Build history of the part. All positions in model axes, mm. A direction names the side the tool comes from. Give positions to 0.01 mm unless a question says otherwise; leave off trailing zeros. Write each loop counter-clockwise with the first axis right and the second up, starting at its lowest first coordinate (ties: lowest second). Pieces come first, ordered by that corner, then holes. Notation, with made-up numbers: M 29.5,43 L 76.5,43 A15 cw 76.5,47 Z; hole C 60.25,4.5 d5. An arc over 180 degrees is marked long. Return JSON: item names as keys, results as strings. Group by question number.
Q1. Band-saw the part on A-A, the plane x = 12.7. Give the cut face in (y, z) (3 decimals).
Q2. Band-saw the part on B-B, the plane y = 25.4. Give the cut face in (x, z) (3 decimals).
Q3. Band-saw the part on D-D, the plane z = 0.25. Count the separate pieces of the cut face and the enclosed holes in it, then the cut area to 3 significant figures.
Q4. Pull direction Y, two halves, no side cores. Call faces 3 (the flat face through (14, 104.775, 0)), 4 (the flat face through (25.4, 66, 0)), 5 (the flat face through (32, 0, 0)): +Y half, -Y half, draft (parallel to the pull), parting line (faces both ways), or undercut.
Q5. Band-saw the part on C-C, the plane x = 38. Give the cut face in (y, z) (3 decimals).
Q6. Flat gauge pins, fed straight in: pin 1 Ø3 at (y, z) = (55.5, 1.5) entering from +X; pin 2 Ø1.9 at (x, z) = (39, 0) entering from +Y. Where does each tip first touch, or does it go through?
Q7. Wall check: probe 1 along Y at (x, z) = (12.7, 1.75) (3 decimals); probe 2 along Y at (x, z) = (50.8, -1.25); probe 3 along Y at (x, z) = (38.1, 1.25). Give the ranges that are in metal, low to high.
Q8. Tool access for faces 1 (the cylindrical face through (29.722, 79.774, -0.044)), 2 (the cylindrical face through (61.59, 1.81, 0.04)): list every direction of +Z, -Z, +X, -X, +Y, -Y with a clear straight run to the whole face (end or side of a thin tool).
from build123d import *

# Parameters (mm, degrees)
SKETCH1_R           = 2.4892
BOSS_EXTRUDE1_DEPTH = 3.175
LPATTERN1_START     = -3.175
LPATTERN1_OUTLINE_R = 2.4892
LPATTERN1_DEPTH     = 6.35
CUT_EXTRUDE1_DEPTH  = 123.679962198
FILLET1_R           = 6.35


# Read off the part's stored shape, not the designer's step: LPattern1
with BuildPart() as part:
    # Sketch1 → Boss-Extrude1 (new, symmetric)
    with BuildSketch(Plane.XY):
        Polygon((0, 0), (0, 104.775), (25.4, 104.775), (63.5, 50.8), (63.5, 0), align=None)
        with Locations((12.7, 85.725)):
            Circle(SKETCH1_R, mode=Mode.SUBTRACT)
        with Locations((12.7, 73.025)):
            Circle(SKETCH1_R, mode=Mode.SUBTRACT)
        with Locations((12.7, 12.7)):
            Circle(SKETCH1_R, mode=Mode.SUBTRACT)
    extrude(amount=BOSS_EXTRUDE1_DEPTH, both=True)

    # LPattern1 outline → LPattern1 (cut)
    with BuildSketch(Plane.XY.offset(LPATTERN1_START)):
        with Locations((50.8, 38.1)):
            Circle(LPATTERN1_OUTLINE_R)
        with Locations((38.1, 38.1)):
            Circle(LPATTERN1_OUTLINE_R)
        with Locations((25.4, 38.1)):
            Circle(LPATTERN1_OUTLINE_R)
        with Locations((12.7, 38.1)):
            Circle(LPATTERN1_OUTLINE_R)
        with Locations((50.8, 25.4)):
            Circle(LPATTERN1_OUTLINE_R)
        with Locations((38.1, 25.4)):
            Circle(LPATTERN1_OUTLINE_R)
        with Locations((25.4, 25.4)):
            Circle(LPATTERN1_OUTLINE_R)
        with Locations((12.7, 25.4)):
            Circle(LPATTERN1_OUTLINE_R)
        with Locations((50.8, 12.7)):
            Circle(LPATTERN1_OUTLINE_R)
        with Locations((38.1, 12.7)):
            Circle(LPATTERN1_OUTLINE_R)
        with Locations((25.4, 12.7)):
            Circle(LPATTERN1_OUTLINE_R)
    extrude(amount=LPATTERN1_DEPTH, mode=Mode.SUBTRACT)

    # Sketch2 → Cut-Extrude1 (cut, through all)
    with BuildSketch(Plane.XY.offset(3.175)):
        Polygon((25.4, 93.763754959), (25.4, 50.8), (55.727356441, 50.8), align=None)
    extrude(amount=-CUT_EXTRUDE1_DEPTH, mode=Mode.SUBTRACT)

    # Fillet1
    fillet1_edges = [part.edges().sort_by_distance(p)[0] for p in [
        (55.727356441, 50.8, 0),
        (25.4, 50.8, 0),
        (25.4, 93.763754959, 0),
        (0, 0, 0),
        (0, 104.775, 0),
        (25.4, 104.775, 0),
        (63.5, 50.8, 0),
        (63.5, 0, 0),
    ]]
    fillet(fillet1_edges, radius=FILLET1_R)


solid = part.part
From the geometry:
{
 "1": {"outline": "M 0,-3.175 L 10.211,-3.175 L 10.211,3.175 L 0,3.175 Z; M 15.189,-3.175 L 22.911,-3.175 L 22.911,3.175 L 15.189,3.175 Z; M 27.889,-3.175 L 35.611,-3.175 L 35.611,3.175 L 27.889,3.175 Z; M 40.589,-3.175 L 70.536,-3.175 L 70.536,3.175 L 40.589,3.175 Z; M 75.514,-3.175 L 83.236,-3.175 L 83.236,3.175 L 75.514,3.175 Z; M 88.214,-3.175 L 104.775,-3.175 L 104.775,3.175 L 88.214,3.175 Z"},
 "2": {"outline": "M 0,-3.175 L 10.211,-3.175 L 10.211,3.175 L 0,3.175 Z; M 15.189,-3.175 L 22.911,-3.175 L 22.911,3.175 L 15.189,3.175 Z; M 27.889,-3.175 L 35.611,-3.175 L 35.611,3.175 L 27.889,3.175 Z; M 40.589,-3.175 L 48.311,-3.175 L 48.311,3.175 L 40.589,3.175 Z; M 53.289,-3.175 L 63.5,-3.175 L 63.5,3.175 L 53.289,3.175 Z"},
 "3": {"separate pieces": "1", "enclosed holes": "15", "area": "4,790 mm^2"},
 "4": {"face 3": "+Y half", "face 4": "undercut", "face 5": "-Y half"},
 "5": {"outline": "M 0,-3.175 L 10.213,-3.175 L 10.213,3.175 L 0,3.175 Z; M 15.187,-3.175 L 22.913,-3.175 L 22.913,3.175 L 15.187,3.175 Z; M 27.887,-3.175 L 35.613,-3.175 L 35.613,3.175 L 27.887,3.175 Z; M 40.587,-3.175 L 50.8,-3.175 L 50.8,3.175 L 40.587,3.175 Z; M 75.914,-3.175 L 86.925,-3.175 L 86.925,3.175 L 75.914,3.175 Z"},
 "6": {"pin 1": "stops at x = 61.24", "pin 2": "stops at y = 86.85"},
 "7": {"probe 1": "y = 0 to 10.211, 15.189 to 22.911, 27.889 to 35.611, 40.589 to 70.536, 75.514 to 83.236, 88.214 to 104.775", "probe 2": "y = 0 to 10.21, 15.19 to 22.91, 27.89 to 35.61, 40.59 to 68.79", "probe 3": "y = 0 to 10.21, 15.19 to 22.91, 27.89 to 35.61, 40.59 to 50.8, 75.77 to 86.78"},
 "8": {"face 1": "+Z, -Z", "face 2": "+Z, -Z, +X, -Y"}
}
